Design review of the part shown in the three views and the two pictorial views. Dimensions are in mm from the part's minimum x, y and z. A direction names the side the tool comes from. Coordinates: 2 decimals unless noted, no trailing zeros. Write each loop counter-clockwise with the first axis right and the second up, starting at its lowest first coordinate (ties: lowest second). Pieces come first, ordered by that corner, then holes. Notation, with made-up numbers: (63.25, 82) - (92.25, 82) arc R30 ccw to (92.25, 121) - close; hole circle Ø3 at (71, 86.25). An arc over 180 degrees is marked (long way). Write each question's results on one line, items separated by ' | '.
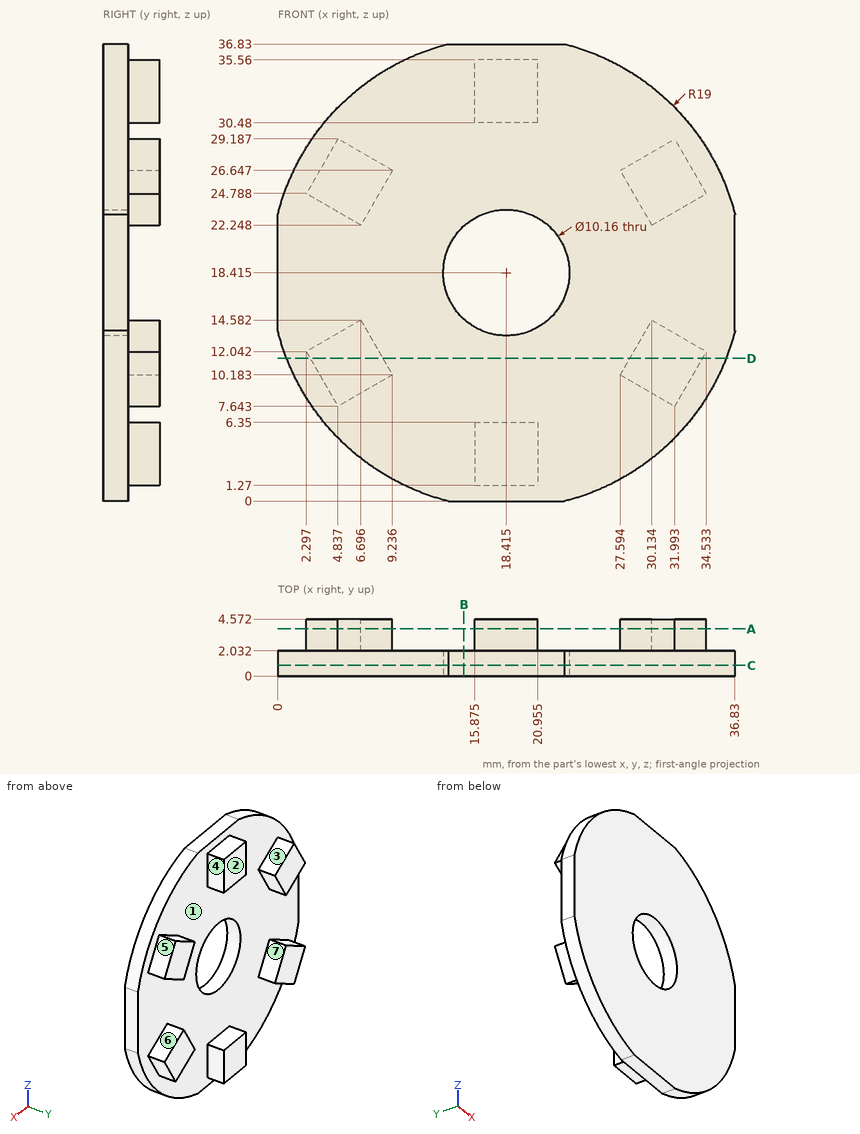
Q1. Take a section at B-B on x = 15. State the section outline as (y, z) points.
Results found:
outline: (0, 0) - (2.03, 0) - (2.03, 14.65) - (0, 14.65) - close; (0, 22.18) - (2.03, 22.18) - (2.03, 36.83) - (0, 36.83) - close
Q2. Take a section at D-D on z = 11.5. State the section outline as (x, y) points.
Results found:
outline: (0.72, 0) - (36.11, 0) - (36.11, 2.03) - (34.22, 2.03) - (34.22, 4.57) - (28.35, 4.57) - (28.35, 2.03) - (8.48, 2.03) - (8.48, 4.57) - (2.61, 4.57) - (2.61, 2.03) - (0.72, 2.03) - close
Q3. Take a section at A-A on y = 3.8. State how many separate pieces and enclosed holes the cut face has, plus the area to 3 significant figures.
Results found:
separate pieces: 6 | enclosed holes: 0 | area: 155 mm2
Q4. Wall thickness on line 1 along Y through (x, z) = (26, 34.5); line 2 along Z through (x, y) = (17, 0.5) (1 decimal); line 3 along X through (y, z) = (2.35, 6) (1 decimal): over which ranges is each line inside the solid? List them lowest first. Write a range as from..to.
Results found:
line 1: 0..2.03 | line 2: 0..13.5, 23.3..36.8 | line 3: 15.9..21
Q5. For the marked faces 4, 5, 6 and 7, list the 3-axis set-ups (+Z, -Z, +X, -X, +Y, -Y) from which the entire face can be reached by the end or side of a thin tool; tool diameter is ignored.
Results found:
face 4: +Z, -Z, +X, +Y | face 5: +Z, +X, +Y | face 6: +X, +Y | face 7: +Y
Q6. For pin 1 (1.3 mm diameter, centred on x = 18.5, y = 4, fed in from +Z); pin 2 (0.8 mm diameter, centred on y = 4, z = 2.5, fed in from -X) (3 decimals); pin 3 (9 mm diameter, centred on x = 18.415, z = 18.415, fed in from -Y); pin 4 (8 mm diameter, centred on x = 7, z = 16, fed in from -Y), all flat-tipped, find the tip position at first contact; note any pin that passes through.
Results found:
pin 1: z = 35.56 | pin 2: x = 15.875 | pin 3: through | pin 4: y = 0
Q7. Mouldability with a two-part tool opening along Z and no side actions: class the marked faces 1, 2 and 3 as pulls with the +Z half, pulls with the -Z half, needs draft (parallel to the pull), parting line crosses it, or undercut.
Results found:
face 1: undercut | face 2: needs draft | face 3: pulls with the +Z half
Q8. Take a section at C-C on y = 0.85. State the section outline as (x, z) points (1 decimal).
Results found:
outline: (0, 13.7) arc R19 ccw to (13.7, 0) - (23.1, 0) arc R19 ccw to (36.8, 13.7) - (36.8, 23.1) arc R19 ccw to (23.1, 36.8) - (13.7, 36.8) arc R19 ccw to (0, 23.1) - close; hole circle Ø10.2 at (18.4, 18.4)
